Input: part model. Units: mm. Frame: model coordinates. A direction names the side the tool comes from. Give positions to 0.01 mm unless a question says otherwise; leave off trailing zeros. Order: outer loops, then holes, each group sorted by start corner. A loop starts at its lowest first (then second) coordinate and runs counter-clockwise, first axis right, second up. Notation, with made-up numbers: (43.25, 3.25) -> (101.25, 3.25) arc R19 cw to (101.25, 31.25) -> close; hole circle Ø8 at (23.25, -16). An arc over 180 degrees is marked (long way). Use a Markdown table: item, result. Add a question column.
Autodesk Inventor part; units mm, degrees
ref_plane "YZ Plane" through (0, 0, 0) normal (1, 0, 0) x (0, 1, 0)
ref_plane "XZ Plane" through (0, 0, 0) normal (0, 1, 0) x (-1, 0, 0)
ref_plane "XY Plane" through (0, 0, 0) normal (0, 0, 1) x (1, 0, 0)
sketch "Sketch1" plane through (0, 0, 0) normal (0, 0, 1) x (1, 0, 0)
  line L0 (88.9, 0) -> (-12.7, 101.6)
  line L1 (-12.7, 101.6) -> (-12.7, -101.6)
  line L2 (-12.7, -101.6) -> (88.9, 0)
  line L3 (-12.7, 0) -> (88.9, 0)
  line L4 (57.4343, 183.898) -> (-323.5657, 183.898)
  line L5 (-323.5657, 183.898) -> (-323.5657, -183.898)
  line L6 (-323.5657, -183.898) -> (57.4343, -183.898)
  line L7 (57.4343, -183.898) -> (57.4343, 183.898)
  line L8 (57.4343, 183.898) -> (-323.5657, -183.898) construction
  line L9 (-323.5657, 183.898) -> (57.4343, -183.898) construction
  circle A0 centre (6.35, 38.1) radius 2.1844
  circle A1 centre (-6.35, 38.1) radius 2.1844
  circle A2 centre (-6.35, -38.1) radius 2.1844
  circle A3 centre (6.35, -38.1) radius 2.1844
  circle A4 centre (6.35, 0) radius 2.1844
  circle A5 centre (6.35, 88.9) radius 2.1844
  circle A6 centre (6.35, 50.8) radius 2.1844
  circle A7 centre (6.35, -50.8) radius 2.1844
  circle A8 centre (-6.35, 0) radius 2.1844
  circle A9 centre (-6.35, 38.1) radius 6.35
  circle A10 centre (-6.35, -38.1) radius 6.35
  line L10 (3.175, -85.725) -> (3.175, -44.45)
  line L11 (3.175, -44.45) -> (-11.204, -44.45)
  line L12 (-10.742, 44.45) -> (3.175, 44.45)
  line L13 (3.175, 44.45) -> (3.175, 85.725)
  point P0 (0, 0)
  point P1 (-133.0657, 0)
  point P2 (57.4343, 31.4657)
  point P3 (-6.35, 44.45)
  point P4 (-12.7, 38.1)
  point P5 (-12.7, -38.1)
  point P6 (-6.35, -44.45)
  point P7 (57.4343, -31.4657)
  dimension "d0" = 101.6
  dimension "d2" = 381
  dimension "d4" = 12.7
  dimension "d5" = 12.7
  dimension "d6" = 3.175
  dimension "d7" = 3.175
extrude "Extrusion1" add sketch "Sketch1" along normal blind 5.08 contours L0 L7 L3 A4 A8 L1 A9 L12 L13 | A9 | L7 L2 L10 L11 A10 L1 L3 A8 A4 | A10
chamfer "Chamfer1" distance 6.35 angle 45 2 edges at (3.175, 44.45, 2.54) (3.175, -44.45, 2.54)
fillet "Fillet1" radius 3.175 4 edges at (3.175, 85.725, 2.54) (3.175, -85.725, 2.54) (57.4343, 31.4657, 2.54) (57.4343, -31.4657, 2.54)
properties part number "wedge"
Q1. Ray query, line 1 (Y direction, x = -6.35, z = 2.65); line 2 (X direction, y = 0, z = 1.95); line 3 (Y direction, x = 6.35, z = 3.6). Return the intervals inside material, ascending.
Q2. Section query A-A (z = 1.4). Give the number of separate pieces and of enclosed holes in the cut face, plus the area to 3 significant figures.
Q3. Section query B-B (x = 44). Return loops of the section in (y, z).
Q4. Section query C-C (y = 55.5). Return loops of the section in (x, z) (3 decimals).
Q5. Access query for faces 4 (the flat face through (-5, 44.45, 3)), 5 (the flat face through (32.9, 56, 2.5)), 6 (the flat face through (-5, -44.45, 3)). Directions: +Z, -Z, +X, -X, +Y, -Y. A direction counts if a zero-diameter tool reaches every point of the face in a straight line with its end or side. Return the directions, or none.
Q6. Draft query along Y for faces 1 (the cylindrical face through (7.524, -39.942, 2.504)), 2 (the flat face through (57.434, 0, 3)), 3 (the cylindrical face through (-10.79, -42.64, 2.5)). Return one class per face: +Y half, -Y half, draft (parallel to the pull), parting line (faces both ways), or undercut.
Q7. First-contact query: pin 1 (3 mm diameter, centred on x = 17.5, z = 4, fed in from +Y); pin 2 (1 mm diameter, centred on x = -4.5, z = 3, fed in from +Y); pin 3 (1.5 mm diameter, centred on y = -59.5, z = 1.5, fed in from -X) (3 decimals). Flat tips, straight axial feed; report the tip coordinate or a pass-through.
Solution:
| question | item | result |
|---|---|---|
| 1 | line 1 | y = -44.45 to -40.28, -35.92 to -2.18, 2.18 to 35.92, 40.28 to 44.45 |
| 1 | line 2 | x = -12.7 to -8.53, -4.17 to 4.17, 8.53 to 57.43 |
| 1 | line 3 | y = -81.23 to -52.98, -48.62 to -40.28, -35.92 to -2.18, 2.18 to 35.92, 40.28 to 48.62, 52.98 to 81.23 |
| 2 | separate pieces | 1 |
| 2 | enclosed holes | 8 |
| 2 | area | 7,650 mm² |
| 3 | outline | (-44.9, 0) -> (44.9, 0) -> (44.9, 5.08) -> (-44.9, 5.08) -> close |
| 4 | outline | (3.175, 0) -> (33.4, 0) -> (33.4, 5.08) -> (3.175, 5.08) -> close |
| 5 | face 4 | +Z, -Z, -X, +Y |
| 5 | face 5 | +Z, -Z, +X, +Y |
| 5 | face 6 | +Z, -Z, -X, -Y |
| 6 | face 1 | undercut |
| 6 | face 2 | draft |
| 6 | face 3 | -Y half |
| 7 | pin 1 | stops at y = 72.9 |
| 7 | pin 2 | stops at y = 44.45 |
| 7 | pin 3 | stops at x = 3.175 |
